Design review of the part built by this model. Coordinates are the model's own, in mm. A direction names the side the tool comes from. Coordinates: 2 decimals unless noted, no trailing zeros. Write each loop counter-clockwise with the first axis right and the second up, starting at its lowest first coordinate (ties: lowest second). Pieces come first, ordered by that corner, then holes. Notation, with made-up numbers: M -14,-29 L 41,-29 A16 cw 41,-4 Z; hole C 53.25,28 d6. An arc over 180 degrees is marked long. Write item = value, one per line.
```python
from build123d import *

# Parameters (mm, degrees)
SKETCH1_W           = 37
SKETCH1_H           = 37
BOSS_EXTRUDE1_DEPTH = 1637.5
SKETCH2_W           = 10
SKETCH2_H           = 20
CUT_EXTRUDE1_DEPTH  = 40
SKETCH3_W           = 21
SKETCH3_H           = 2
CUT_EXTRUDE2_DEPTH  = 20
SKETCH4_W           = 8.1
SKETCH4_H           = 41
CUT_EXTRUDE3_DEPTH  = 1639.476807892
CUT_EXTRUDE4_DEPTH  = 20
SKETCH6_W           = 20
SKETCH6_H           = 20
CUT_EXTRUDE5_DEPTH  = 20
SKETCH7_R           = 10
CUT_EXTRUDE6_DEPTH  = 1639.476807892
SKETCH8_R           = 10
CUT_EXTRUDE7_DEPTH  = 1639.476807892
SKETCH9_W           = 10
SKETCH9_H           = 55
CUT_EXTRUDE8_DEPTH  = 10


with BuildPart() as part:
    # Sketch1 → Boss-Extrude1 (new body)
    with BuildSketch(Plane(origin=(0, 0, 0), x_dir=(1, 0, 0), z_dir=(0, 1, 0))):
        with BuildLine():
            Line((0.5, 0), (39.5, 0))
            ThreePointArc((39.5, 0), (39.853553391, 0.146446609), (40, 0.5))
            Line((40, 0.5), (40, 39.5))
            ThreePointArc((40, 39.5), (39.853553391, 39.853553391), (39.5, 40))
            Line((39.5, 40), (0.5, 40))
            ThreePointArc((0.5, 40), (0.146446609, 39.853553391), (0, 39.5))
            Line((0, 39.5), (0, 0.5))
            ThreePointArc((0, 0.5), (0.146446609, 0.146446609), (0.5, 0))
        make_face()
        with Locations((20, 20)):
            Rectangle(SKETCH1_W, SKETCH1_H, mode=Mode.SUBTRACT)
    extrude(amount=BOSS_EXTRUDE1_DEPTH)

    # Sketch2 → Cut-Extrude1 (cut)
    with BuildSketch(Plane.XY.offset(-40)):
        with Locations((35, 1627.5)):
            Rectangle(SKETCH2_W, SKETCH2_H)
        with Locations((5, 1627.5)):
            Rectangle(SKETCH2_W, SKETCH2_H)
    extrude(amount=CUT_EXTRUDE1_DEPTH, mode=Mode.SUBTRACT)

    # Sketch3 → Cut-Extrude2 (cut)
    with BuildSketch(Plane(origin=(40, 0, 0), x_dir=(0, 0, -1), z_dir=(1, 0, 0))):
        with Locations((29.5, 1534)):
            Rectangle(SKETCH3_W, SKETCH3_H)
        with Locations((29.5, 1496)):
            Rectangle(SKETCH3_W, SKETCH3_H)
    extrude(amount=-CUT_EXTRUDE2_DEPTH, mode=Mode.SUBTRACT)

    # Sketch4 → Cut-Extrude3 (cut, through all)
    with BuildSketch(Plane.ZY):
        with Locations((-4.05, 20.5)):
            Rectangle(SKETCH4_W, SKETCH4_H)
        with Locations((-35.95, 20.5)):
            Rectangle(SKETCH4_W, SKETCH4_H)
    extrude(amount=-CUT_EXTRUDE3_DEPTH, mode=Mode.SUBTRACT)

    # Sketch5 → Cut-Extrude4 (cut)
    with BuildSketch(Plane(origin=(40, 0, -40), x_dir=(0, 0, 1), z_dir=(-1, 0, 0))):
        Polygon((40, 190.5), (20, 190.5), (20, 231), (30, 231), (30, 211), (40, 211), align=None)
        Polygon((40, 380.5), (20, 380.5), (20, 421), (30, 421), (30, 401), (40, 401), align=None)
        Polygon((40, 570.5), (20, 570.5), (20, 611), (30, 611), (30, 591), (40, 591), align=None)
        Polygon((40, 760.5), (20, 760.5), (20, 801), (30, 801), (30, 781), (40, 781), align=None)
    extrude(amount=CUT_EXTRUDE4_DEPTH, mode=Mode.SUBTRACT)

    # Sketch6 → Cut-Extrude5 (cut)
    with BuildSketch(Plane(origin=(0, 0, -40), x_dir=(-1, 0, 0), z_dir=(0, 0, -1))):
        with Locations((-30, 1033)):
            Rectangle(SKETCH6_W, SKETCH6_H)
    extrude(amount=-CUT_EXTRUDE5_DEPTH, mode=Mode.SUBTRACT)

    # Sketch7 → Cut-Extrude6 (cut, through all)
    with BuildSketch(Plane(origin=(40, 0, 0), x_dir=(0, 0, -1), z_dir=(1, 0, 0))):
        with Locations((20, 1577.5)):
            Circle(SKETCH7_R)
        with Locations((20, 1227.5)):
            Circle(SKETCH7_R)
    extrude(amount=-CUT_EXTRUDE6_DEPTH, mode=Mode.SUBTRACT)

    # Sketch8 → Cut-Extrude7 (cut, through all)
    with BuildSketch(Plane.XY):
        with Locations((25, 1467.5)):
            Circle(SKETCH8_R)
        with Locations((25, 1197.5)):
            Circle(SKETCH8_R)
        with Locations((25, 927.5)):
            Circle(SKETCH8_R)
        with Locations((25, 151)):
            Circle(SKETCH8_R)
        with Locations((25, 331)):
            Circle(SKETCH8_R)
        with Locations((25, 511)):
            Circle(SKETCH8_R)
        with Locations((25, 691)):
            Circle(SKETCH8_R)
        with Locations((25, 871)):
            Circle(SKETCH8_R)
    extrude(amount=-CUT_EXTRUDE7_DEPTH, mode=Mode.SUBTRACT)

    # Sketch9 → Cut-Extrude8 (cut)
    with BuildSketch(Plane(origin=(40, 0, 0), x_dir=(0, 0, -1), z_dir=(1, 0, 0))):
        with Locations((18, 508.5)):
            Rectangle(SKETCH9_W, SKETCH9_H)
    extrude(amount=-CUT_EXTRUDE8_DEPTH, mode=Mode.SUBTRACT)


solid = part.part
```
Q1. For P1, Ø1.2, axis at y = 581.5, z = -1, coming from the +X side; P2, Ø1.6, axis at y = 1624, z = -39.5, coming from the -X side; P3, Ø11, axis at x = 29, z = -3.5, coming from the -Y side, all flat-tipped, find the tip position at first contact; note any pin that passes through.
Check result:
P1 = 20
P2 = 10
P3 = 41
Q2. Consider section A-A, the plane y = 640. State the section outline as (x, z) points.
Check result:
outline = M 0,-39.5 A0.5 ccw 0.5,-40 L 39.5,-40 A0.5 ccw 40,-39.5 L 40,-0.5 A0.5 ccw 39.5,0 L 0.5,0 A0.5 ccw 0,-0.5 Z; hole M 1.5,-38.5 L 38.5,-38.5 L 38.5,-1.5 L 1.5,-1.5 Z
Q3. Wall thickness on line 1 (Z direction, x = 0.65, y = 1227.5); line 2 (X direction, y = 871, z = -0.3); line 3 (X direction, y = 257.5, z = -25): over which ranges is each line inside the solid? List them lowest first.
Check result:
line_1 = -40 to -30, -10 to 0
line_2 = 0.04 to 15, 35 to 39.96
line_3 = 0 to 1.5, 38.5 to 40
Q4. The part is to be moulded in two halves that separate along Z. For faces 1 (the flat face through (38.5, 797, -24)), 2 (the flat face through (0, 797, -20)), 3 (the flat face through (20, 828, 0)), say which applies: +Z half, -Z half, draft (parallel to the pull), parting line (faces both ways), or undercut.
Check result:
face_1 = undercut
face_2 = draft
face_3 = +Z half
Q5. Machinability: for faces 4 (the flat face through (20, 828, -38.5)), 5 (the flat face through (40, 797, -24)), which of the approach directions +Z, -Z, +X, -X, +Y, -Y give a long, thin tool a straight path to every point of the face, cutting with its end or side? Answer none if there is none.
Check result:
face_4 = +Y, -Y
face_5 = +Z, -Z, +X, +Y, -Y
